Source: CAD feature listing. Evaluate the final solid. Frame: model axes, mm. Face numbers are marked on the shaded views. Round coordinates to 2 decimals unless told otherwise and drop trailing zeros. Write each loop counter-clockwise with the first axis right and the second up, starting at its lowest first coordinate (ties: lowest second). Pieces come first, ordered by that corner, then holes.
```python
from build123d import *

# Parameters (mm, degrees)
F0_R     = 65
F0_R_2   = 55
F1_DEPTH = 26
F2_SIZE  = 5
F3_SIZE  = 2


with BuildPart() as f1:
    # F0 (on Right) → F1 (new body, symmetric)
    with BuildSketch(Plane.YZ):
        Circle(F0_R)
        Circle(F0_R_2, mode=Mode.SUBTRACT)
    extrude(amount=F1_DEPTH, both=True)

    # F2
    f2_edges = [f1.edges().sort_by_distance(p)[0] for p in [
        (-26, -55, 0),
    ]]
    chamfer(f2_edges, length=F2_SIZE)

    # F3
    f3_edges = [f1.edges().sort_by_distance(p)[0] for p in [
        (-26, -65, 0),
        (26, -65, 0),
        (26, -55, 0),
    ]]
    chamfer(f3_edges, length=F3_SIZE)


solid = f1.part
```
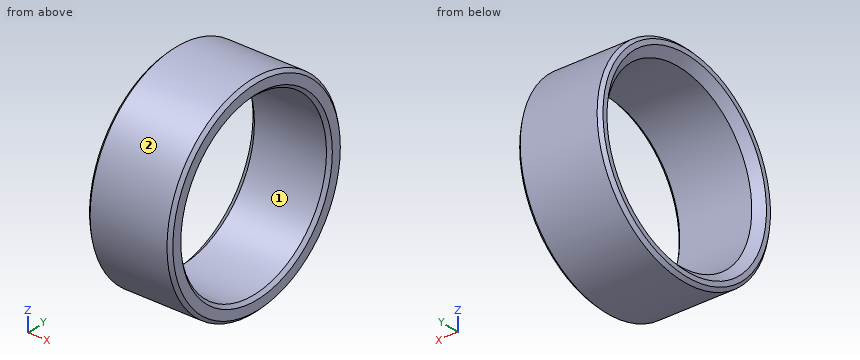
Q1. Line query: line 1 (Z direction, x = 3, y = 0); line 2 (Y direction, x = 24, z = -26); line 3 (Z direction, x = -9, y = -42). Output: solid intervals per line, ascending.
Q2. Mould query, pull axis Z, two halves, no side actions, for the marked faces 1 and 2. Classes: pulls with the +Z half, pulls with the -Z half, needs draft (parallel to the pull), parting line crosses it, or undercut.
Q3. Section query C-C, the plane x = 22. Output: boundary loops of the cut face in (y, z).
Q4. Pin query (flat end, axial travel): P1, Ø2, axis at x = -2, z = -35.5, coming from the -Y side; P2, Ø3, axis at x = -15, y = 26.5, coming from the -Z side; P3, Ø1.5, axis at x = -9.5, z = 35, coming from the -Y side. Return the tip coordinate at first contact, or that it passes through.
Q5. Section query A-A, the plane z = 0. Output: boundary loops of the cut face in (x, y), and give its area (3 significant figures).
Filled in:
1. line 1: z = -65 to -55, 55 to 65
1. line 2: y = -59.57 to -48.47, 48.47 to 59.57
1. line 3: z = -49.61 to -35.51, 35.51 to 49.61
2. face 1: undercut
2. face 2: parting line crosses it
3. outline: circle Ø130 at (0, 0); hole circle Ø110 at (0, 0)
4. P1: stops at y = -55.09
4. P2: stops at z = -60
4. P3: stops at y = -55.24
5. outline: (-26, -63) - (-24, -65) - (24, -65) - (26, -63) - (26, -57) - (24, -55) - (-21, -55) - (-26, -60) - close; (-26, 60) - (-21, 55) - (24, 55) - (26, 57) - (26, 63) - (24, 65) - (-24, 65) - (-26, 63) - close
5. area: 1,000 mm2
